from build123d import *

# Parameters (mm, degrees)
SKETCH1_R           = 7
BOSS_EXTRUDE1_DEPTH = 44
SKETCH2_R           = 5.5
CUT_EXTRUDE1_DEPTH  = 99.636339936
CUT_EXTRUDE2_START  = -19
CUT_EXTRUDE2_DEPTH  = 19
CUT_EXTRUDE3_DEPTH  = 24
CUT_EXTRUDE4_DEPTH  = 7
CUT_EXTRUDE5_DEPTH  = 25


with BuildPart() as part:
    # Sketch1 → Boss-Extrude1 (new body)
    with BuildSketch(Plane.XY):
        with BuildLine():
            ThreePointArc((-40.404910175, -1.633500031), (-37.139674394, -2.846913799), (-35.459271434, -5.898205914))
            ThreePointArc((-35.459271434, -5.898205914), (-33.122441231, -13.749172092), (-28.683469034, -20.633500031))
            Line((-28.683469034, -20.633500031), (-22.980449087, -20.633500031))
            Line((-22.980449087, -20.633500031), (6.019550913, 13.366499969))
            Line((6.019550913, 13.366499969), (6.019550913, 32.366499969))
            Line((6.019550913, 32.366499969), (1.019550913, 37.366499969))
            Line((1.019550913, 37.366499969), (-22.980449087, 37.366499969))
            ThreePointArc((-22.980449087, 37.366499969), (-28.648710625, 28.077944899), (-39.256864445, 25.654410975))
            Line((-39.256864445, 25.654410975), (-65.980449087, 30.366499969))
            Line((-65.980449087, 30.366499969), (-72.980449087, 30.366499969))
            Line((-72.980449087, 30.366499969), (-79.980449087, 23.366499969))
            Line((-79.980449087, 23.366499969), (-79.980449087, 5.366499969))
            Line((-79.980449087, 5.366499969), (-72.980449087, -1.633500031))
            Line((-72.980449087, -1.633500031), (-40.404910175, -1.633500031))
        make_face()
        with Locations((-65.980449087, 12.366499969)):
            Circle(SKETCH1_R, mode=Mode.SUBTRACT)
    extrude(amount=BOSS_EXTRUDE1_DEPTH)

    # Sketch2 → Cut-Extrude1 (cut, through all)
    with BuildSketch(Plane.XY.offset(44)):
        with Locations((-7.980449087, 23.366499969)):
            Circle(SKETCH2_R)
    extrude(amount=-CUT_EXTRUDE1_DEPTH, mode=Mode.SUBTRACT)

    # Sketch3 → Cut-Extrude2 (cut)
    with BuildSketch(Plane.XY.offset(44).offset(CUT_EXTRUDE2_START)):
        Polygon((-45.980449087, 26.839960355), (-45.980449087, -1.633500031), (-72.980449087, -1.633500031), (-79.980449087, 5.366499969), (-79.980449087, 23.366499969), (-72.980449087, 30.366499969), (-65.980449087, 30.366499969), align=None)
        with BuildLine():
            Line((-40.404910175, -1.633500031), (-6.774566734, -1.633500031))
            Line((-6.774566734, -1.633500031), (-22.980449087, -20.633500031))
            Line((-22.980449087, -20.633500031), (-28.683469034, -20.633500031))
            ThreePointArc((-28.683469034, -20.633500031), (-33.122441231, -13.749172092), (-35.459271434, -5.898205914))
            ThreePointArc((-35.459271434, -5.898205914), (-37.139674394, -2.846913799), (-40.404910175, -1.633500031))
        make_face()
    extrude(amount=CUT_EXTRUDE2_DEPTH, mode=Mode.SUBTRACT)

    # Sketch7 → Cut-Extrude3 (cut)
    with BuildSketch(Plane(origin=(0, 0, 12), x_dir=(-1, 0, 0), z_dir=(0, 0, -1))):
        with BuildLine():
            Line((-6.019550913, 13.366499969), (4.215743204, 1.366499969))
            ThreePointArc((4.215743204, 1.366499969), (21.210918642, 10.417084234), (32.200340902, 26.227892629))
            ThreePointArc((32.200340902, 26.227892629), (26.041094158, 30.514775107), (22.980449087, 37.366499969))
            Line((22.980449087, 37.366499969), (-1.019550913, 37.366499969))
            Line((-1.019550913, 37.366499969), (-6.019550913, 32.366499969))
            Line((-6.019550913, 32.366499969), (-6.019550913, 13.366499969))
        make_face()
    extrude(amount=-CUT_EXTRUDE3_DEPTH, mode=Mode.SUBTRACT)

    # Sketch8 → Cut-Extrude4 (cut)
    with BuildSketch(Plane.XY.offset(44)):
        with BuildLine():
            Line((-44.980449087, 25.648206762), (-44.980449087, -0.633500031))
            Line((-44.980449087, -0.633500031), (-7.235972791, -0.633500031))
            Line((-7.235972791, -0.633500031), (5.019550913, 13.735045001))
            Line((5.019550913, 13.735045001), (5.019550913, 31.952286406))
            Line((5.019550913, 31.952286406), (0.605337351, 36.366499969))
            Line((0.605337351, 36.366499969), (-22.144406347, 36.366499969))
            ThreePointArc((-22.144406347, 36.366499969), (-28.419495692, 27.018587194), (-39.430512622, 24.669603222))
            Line((-39.430512622, 24.669603222), (-44.980449087, 25.648206762))
        make_face()
    extrude(amount=-CUT_EXTRUDE4_DEPTH, mode=Mode.SUBTRACT)

    # Sketch12 → Cut-Extrude5 (cut)
    with BuildSketch(Plane.XY.offset(37)):
        with BuildLine():
            Line((-7.235972791, -0.633500031), (-5.99360134, 0.823073394))
            ThreePointArc((-5.99360134, 0.823073394), (-22.117044704, 9.886135078), (-32.783766787, 24.996580242))
            ThreePointArc((-32.783766787, 24.996580242), (-36.088777964, 24.459836681), (-39.430512622, 24.669603222))
            Line((-39.430512622, 24.669603222), (-44.980449087, 25.648206762))
            Line((-44.980449087, 25.648206762), (-44.980449087, -0.633500031))
            Line((-44.980449087, -0.633500031), (-7.235972791, -0.633500031))
        make_face()
    extrude(amount=-CUT_EXTRUDE5_DEPTH, mode=Mode.SUBTRACT)


solid = part.part
Can you work these out from the model? Positions are in its coordinate system, mm. A direction names the side the tool comes from. Coordinates: 2 decimals unless noted, no trailing zeros. Write each loop counter-clockwise with the first axis right and the second up, starting at its lowest first coordinate (ties: lowest second). Pieces come first, ordered by that corner, then holes. Notation, with made-up numbers: M -13.5,14 L -5.5,14 A23 ccw -5.5,23 Z; hole C 1,-24 d4. An arc over 180 degrees is marked long. Use one line per item in the form item = value.
Q1. If we section it at B-B (y = 33.5): Write out the boundary of the cut face in (x, z), then the cut area to 3 significant figures.
Model answer:
outline = M -24.15,0 L 4.89,0 L 4.89,12 L -24.15,12 Z; M -24.15,36 L 4.89,36 L 4.89,44 L 3.47,44 L 3.47,37 L -23.05,37 L -23.05,44 L -24.15,44 Z
area = 395 mm^2
Q2. If we section it at D-D (z = 17.5): Write out the boundary of the cut face in (x, y).
Model answer:
outline = M -79.98,5.37 L -72.98,-1.63 L -40.4,-1.63 A5 cw -35.46,-5.9 A29 ccw -28.68,-20.63 L -22.98,-20.63 L -4.22,1.37 A41 cw -32.2,26.23 A14 cw -39.26,25.65 L -65.98,30.37 L -72.98,30.37 L -79.98,23.37 Z; hole C -65.98,12.37 d14; hole M -44.98,-0.63 L -7.24,-0.63 L -5.99,0.82 A42 cw -32.78,25 A15 cw -39.43,24.67 L -44.98,25.65 Z
Q3. For faces 4 (the flat face through (-45.98, 13, 34)), 5 (the cylindrical face through (-21.01, 10.24, 23.83)), 6 (the flat face through (3.555, 34.831, 5.916)), 7 (the flat face through (-11, 36.366, 41)), 8 (the cylindrical face through (-5.44, 18.49, 36.51)), which set-ups out of +Z, -Z, +X, -X, +Y, -Y let a thin tool reach every point of the face, with its end or its side?
Model answer:
face_4 = +Z, -X, +Y, -Y
face_5 = +X, +Y
face_6 = +Z, -Z, +X, +Y
face_7 = +Z
face_8 = +Z, -Z
Q4. If we section it at C-C (x = -60.5): Write out the boundary of the cut face in (y, z).
Model answer:
outline = M -1.63,0 L 8.01,0 L 8.01,25 L -1.63,25 Z; M 16.72,0 L 29.4,0 L 29.4,25 L 16.72,25 Z
Q5. If we section it at A-A (z = 34): Write out the boundary of the cut face in (x, y).
Model answer:
outline = M -45.98,-1.63 L -6.77,-1.63 L -4.22,1.37 A41 cw -32.2,26.23 A14 cw -39.26,25.65 L -45.98,26.84 Z; hole M -44.98,-0.63 L -7.24,-0.63 L -5.99,0.82 A42 cw -32.78,25 A15 cw -39.43,24.67 L -44.98,25.65 Z
Q6. For P1, Ø5.5, axis at x = -11, z = 42, coming from the -Y side; P2, Ø11, axis at x = -19.5, y = 24, coming from the +Z side; P3, Ø21, axis at y = 12.5, z = 36, coming from the +X side; P4, Ø9.5, axis at y = 5.5, z = 32.5, coming from the -X side, each with a flat end and sliding along its axis, tell me the tip position at first contact or that it passes through.
Model answer:
P1 = -1.63
P2 = 37
P3 = 6.02
P4 = -45.98
Q7. I need wall thicknesses on line 1 along Z through (x, y) = (-15.5, 24); line 2 along Y through (x, z) = (-12, 37.5); line 3 along Y through (x, z) = (-66, 8). Which ranges of each line are inside material? Lowest first, please. Write a range as from..to.
Model answer:
line_1 = 0..12, 36..37
line_2 = -1.63..-0.63, 36.37..37.37
line_3 = -1.63..5.37, 19.37..30.37
Q8. We'd pull the mould along Z, two halves only. Please class faces 1 (the flat face through (-13, 20, 36)), 2 (the cylindrical face through (-5.44, 18.49, 6.08)), 3 (the flat face through (-14, 19, 37)): +Z half, -Z half, draft (parallel to the pull), parting line (faces both ways), or undercut.
Model answer:
face_1 = undercut
face_2 = draft
face_3 = +Z half
